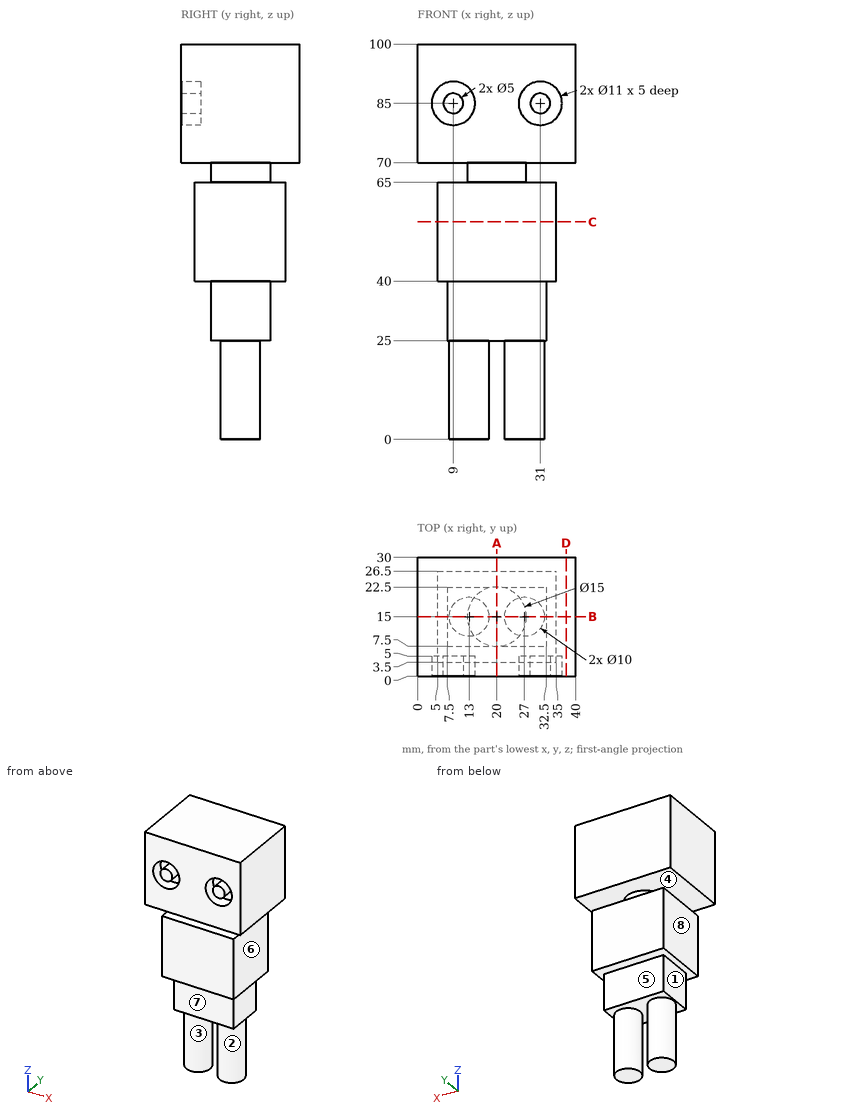
Verification items for this drawing (mm, ordinates from the low corner). A direction names the side the tool comes from. Coordinates: 2 decimals unless noted, no trailing zeros. Loops run counter-clockwise (first coordinate to the right, second up) from the corner with the lowest first, then second, coordinate; pieces in that order, holes last. Notation, with made-up numbers: (-24, 26) -> (-8, 26) arc R21 ccw to (-8, 51) -> close; hole circle Ø3 at (89, 26.25). An arc over 180 degrees is marked (long way). Answer in a Markdown table with one row per item. Add a question column.
1. Section check A-A, the plane x = 20. Enter the section's corners in (y, z).
2. Material ranges on probe 1 along Z at (x, y) = (9, 1.7); probe 2 along Z at (x, y) = (11, 2.75); probe 3 along X at (y, z) = (3, 81), recorded low to high. Write a range as [from, to].
3. Section check C-C, the plane z = 55. Enter the section's corners in (x, y).
4. Draft check along X on the marked faces 1, 2, 3 and 4. Enter one of: +X half, -X half, draft (parallel to the pull), parting line (faces both ways), or undercut.
5. Section check D-D, the plane x = 37.5. Enter the section's corners in (y, z).
6. Depth check by flat-ended pin: P1, Ø7, axis at y = 12, z = 53, coming from the -X side; P2, Ø4.5, axis at y = 14.5, z = 32.5, coming from the -X side; P3, Ø12, axis at x = 23.5, z = 32, coming from the -Y side. Enter the tip coordinate at first touch or a pass-through.
7. Access from +Z, -Z, +X, -X, +Y, -Y to the whole of each face (thin tool, end or side, straight path). Record for the marked faces 5, 6, 7 and 8.
8. Section check B-B, the plane y = 15. Enter the section's corners in (x, z).
Derived:
| question | item | result |
|---|---|---|
| 1 | outline | (0, 70) -> (7.5, 70) -> (7.5, 65) -> (3.5, 65) -> (3.5, 40) -> (7.5, 40) -> (7.5, 25) -> (22.5, 25) -> (22.5, 40) -> (26.5, 40) -> (26.5, 65) -> (22.5, 65) -> (22.5, 70) -> (30, 70) -> (30, 100) -> (0, 100) -> close |
| 2 | probe 1 | z = [70, 79.5], [82.5, 87.5], [90.5, 100] |
| 2 | probe 2 | z = [70, 79.88], [83.5, 86.5], [90.12, 100] |
| 2 | probe 3 | x = [0, 5.23], [12.77, 27.23], [34.77, 40] |
| 3 | outline | (5, 3.5) -> (35, 3.5) -> (35, 26.5) -> (5, 26.5) -> close |
| 4 | face 1 | -X half |
| 4 | face 2 | undercut |
| 4 | face 3 | undercut |
| 4 | face 4 | draft |
| 5 | outline | (0, 70) -> (30, 70) -> (30, 100) -> (0, 100) -> close |
| 6 | P1 | stops at x = 5 |
| 6 | P2 | stops at x = 7.5 |
| 6 | P3 | stops at y = 7.5 |
| 7 | face 5 | -Z, +X, -X, +Y |
| 7 | face 6 | -Z, +X, +Y, -Y |
| 7 | face 7 | -Z, +X, -X, -Y |
| 7 | face 8 | -Z, -X, +Y, -Y |
| 8 | outline | (0, 70) -> (12.5, 70) -> (12.5, 65) -> (5, 65) -> (5, 40) -> (7.5, 40) -> (7.5, 25) -> (8, 25) -> (8, 0) -> (18, 0) -> (18, 25) -> (22, 25) -> (22, 0) -> (32, 0) -> (32, 25) -> (32.5, 25) -> (32.5, 40) -> (35, 40) -> (35, 65) -> (27.5, 65) -> (27.5, 70) -> (40, 70) -> (40, 100) -> (0, 100) -> close |
